Can you work these out from the drawing? Everything is in mm from the part's minimum corner. Give positions to 0.01 mm unless a question says otherwise; leave off trailing zeros. Loops run counter-clockwise (first coordinate to the right, second up) from the corner with the lowest first, then second, coordinate; pieces in that order, holes last. Notation, with made-up numbers: (7.25, 23) - (44.25, 23) arc R25 cw to (44.25, 39) - close; hole circle Ø5 at (66, 40). An arc over 180 degrees is marked (long way). One line per item, written item: value. Start each with the question number.
Q1. I want a section at A-A (y = 5). Please give me the cut outline in (x, z).
Q2. I'm going to push flat-ended pins straight in: P1, Ø2, axis at y = 36.5, z = 7, coming from the -X side; P2, Ø9, axis at x = 16, y = 14.5, coming from the +Z side. Where does each tip first touch, or does it pass through?
Q3. I want a section at D-D (y = 35). Please give me the cut outline in (x, z).
Q4. If I drill on line 1 (Y direction, x = 15, z = 4.75); line 2 (Y direction, x = 5, z = 2.8); line 3 (Z direction, x = 27, y = 20), over which ranges is the centre line in solid material (lowest first)? Write a range as from..to.
Q5. If we mould it in two halves opening along X, with no side actions, what happens to the marked faces 1, 2, 3 and 4? For each: released by +X, released by -X, zero draft, split by the parting line, or undercut.
Q6. I want a section at C-C (z = 3.5). Please give me the cut outline in (x, y), then the cut area to 3 significant figures.
Q7. I want a section at B-B (x = 5). Please give me the cut outline in (y, z).
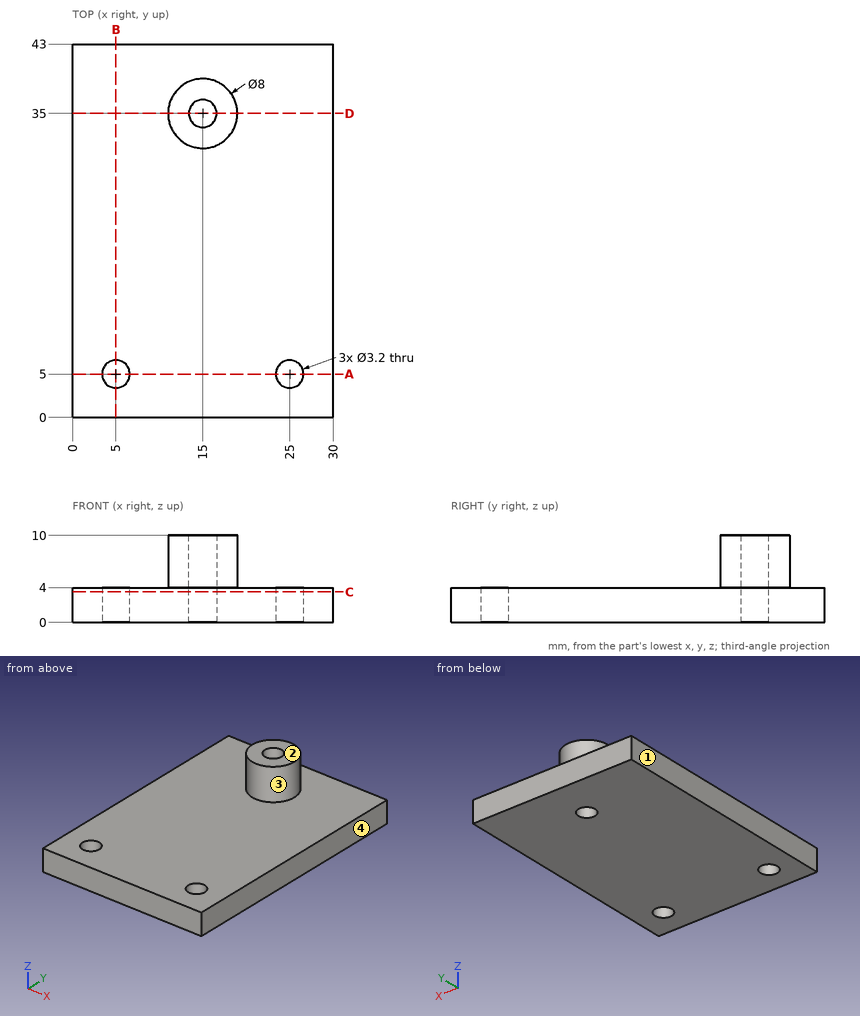
Worked answers:
1. outline: (0, 0) - (3.4, 0) - (3.4, 4) - (0, 4) - close; (6.6, 0) - (23.4, 0) - (23.4, 4) - (6.6, 4) - close; (26.6, 0) - (30, 0) - (30, 4) - (26.6, 4) - close
2. P1: stops at x = 11.03
2. P2: stops at z = 4
3. outline: (0, 0) - (13.4, 0) - (13.4, 10) - (11, 10) - (11, 4) - (0, 4) - close; (16.6, 0) - (30, 0) - (30, 4) - (19, 4) - (19, 10) - (16.6, 10) - close
4. line 1: y = 31..33.4, 36.6..39
4. line 2: y = 0..3.4, 6.6..43
4. line 3: z = 0..4
5. face 1: released by -X
5. face 2: zero draft
5. face 3: split by the parting line
5. face 4: released by +X
6. outline: (0, 0) - (30, 0) - (30, 43) - (0, 43) - close; hole circle Ø3.2 at (5, 5); hole circle Ø3.2 at (15, 35); hole circle Ø3.2 at (25, 5)
6. area: 1,270 mm²
7. outline: (0, 0) - (3.4, 0) - (3.4, 4) - (0, 4) - close; (6.6, 0) - (43, 0) - (43, 4) - (6.6, 4) - close
